Source: CAD feature listing. Evaluate the final solid. Frame: model axes, mm. A direction names the side the tool comes from. Round coordinates to 2 decimals unless told otherwise and drop trailing zeros. Write each loop counter-clockwise with the first axis right and the second up, starting at its lowest first coordinate (ties: lowest second). Pieces come first, ordered by that corner, then holes. Notation, with made-up numbers: M -28,-22 L -10,-22 A18 cw -10,10 Z; hole C -36.5,-16.5 d6. An arc over 180 degrees is marked long. Put each result on its own line as item: value. Start each with the question number.
Autodesk Inventor part; units mm, degrees
ref_plane "YZ Plane" through (0, 0, 0) normal (1, 0, 0) x (0, 1, 0)
ref_plane "XZ Plane" through (0, 0, 0) normal (0, 1, 0) x (-1, 0, 0)
ref_plane "XY Plane" through (0, 0, 0) normal (0, 0, 1) x (1, 0, 0)
sketch "Schizzo3" plane through (0, 0, 0) normal (0, 1, 0) x (-1, 0, 0)
  circle A0 centre (0, 75) radius 2.75
  circle A1 centre (0, -75) radius 2.75
  line L0 (-230, 0) -> (-230, 100)
  line L1 (230, 100) -> (230, 0)
  line L2 (-230, 0) -> (-230, -100)
  line L3 (230, -100) -> (230, 0)
  line L4 (-230, 0) -> (-230, 190)
  line L5 (-220, 200) -> (220, 200)
  line L6 (230, 190) -> (230, 2)
  line L7 (-230, 0) -> (-230, -190)
  line L8 (-220, -200) -> (220, -200)
  line L9 (230, -190) -> (230, 0)
  arc A2 (228, 0) -> (230, 2) centre (228, 2) ccw
  arc A3 (230, 190) -> (220, 200) centre (220, 190) ccw
  arc A4 (220, -200) -> (230, -190) centre (220, -190) ccw
  arc A5 (-230, -190) -> (-220, -200) centre (-220, -190) ccw
  arc A6 (-220, 200) -> (-230, 190) centre (-220, 190) ccw
  point P0 (0, 0)
  point P1 (-230, 200)
  point P2 (-230, -200)
  dimension "d18" = 5.5
  dimension "d21" = 5.5
  dimension "d24" = 460
  dimension "d25" = 460
  dimension "d26" = 100
  dimension "d27" = 200
  dimension "d28" = 200
  dimension "d29" = 2
  dimension "d30" = 10
extrude "Estrusione3" add sketch "Schizzo3" along normal blind 10
sketch "Schizzo4" plane through (0, 10, 0) normal (0, 1, 0) x (1, 0, 0)
  circle A0 centre (0, 0) radius 160.6805
extrude "Estrusione4" add sketch "Schizzo4" along normal blind 10
properties part number "Pedana_Stampa 3D"
(1) Section query C-C (x = -181.5). Return loops of the section in (y, z), and give its area (3 significant figures).
(2) Section query B-B (x = 38.5). Return loops of the section in (y, z).
(3) Contact query for flat-ended pins moving along their axis: P1, Ø2, axis at y = 12, z = -77.5, coming from the -X side; P2, Ø3, axis at y = 13.5, z = 139.5, coming from the +X side; P3, Ø2, axis at y = 14, z = 32.5, coming from the -X side. Output: stop coordinate, or through.
(4) Ray query, line 1 along Z through (x, y) = (0, 4.25); line 2 along Y through (x, z) = (-162.5, 25.5); line 3 along X through (y, z) = (17.75, -34). Return the intervals inside material, ascending.
(5) Access query for faces 1 (the flat face through (-230, 5, 3)), 2 (the flat face through (157, 10, 47)). Directions: +Z, -Z, +X, -X, +Y, -Y. A direction counts if a zero-diameter tool reaches every point of the face in a straight line with its end or side. Return the directions, or none.
(6) Section query A-A (z = 0). Return loops of the section in (x, y), and give its area (3 significant figures).
Entries:
1. outline: M 0,-200 L 10,-200 L 10,200 L 0,200 Z
1. area: 4,000 mm2
2. outline: M 0,-200 L 10,-200 L 10,-156 L 20,-156 L 20,156 L 10,156 L 10,200 L 0,200 Z
3. P1: x = -141.3
3. P2: x = 82.31
3. P3: x = -157.56
4. line 1: -200 to -77.75, -72.25 to 72.25, 77.75 to 200
4. line 2: 0 to 10
4. line 3: -157.04 to 157.04
5. face 1: +Z, -Z, -X, +Y, -Y
5. face 2: +Y
6. outline: M -230,0 L 230,0 L 230,10 L 160.68,10 L 160.68,20 L -160.68,20 L -160.68,10 L -230,10 Z
6. area: 7,810 mm2
